from build123d import *

# Parameters (mm, degrees)
F1_W     = 76
F1_H     = 72
F2_DEPTH = 1.2
F3_R     = 30
F5_DEPTH = 28.8


with BuildPart() as f2:
    # F1 (on offset) → F2 (new body)
    with BuildSketch(Plane.XY.offset(30)):
        with Locations((0, 36)):
            Rectangle(F1_W, F1_H)
    extrude(amount=-F2_DEPTH)

    # F3
    f3_edges = [f2.edges().sort_by_distance(p)[0] for p in [
        (-38, 72, 29.4),
        (38, 72, 29.4),
    ]]
    fillet(f3_edges, radius=F3_R)

    # F4 (on face) → F5 (join, through all)
    with BuildSketch(Plane(origin=(0, 0, 28.8), x_dir=(1, 0, 0), z_dir=(0, 0, -1))):
        Polygon((5, -20), (18, -20), (18, -10), (-18, -10), (-18, -20), (-5, -20), (-5, -52), (5, -52), align=None)
        Polygon((3, -18), (3, -50), (-3, -50), (-3, -18), (-16, -18), (-16, -12), (16, -12), (16, -18), align=None, mode=Mode.SUBTRACT)
    extrude(amount=F5_DEPTH)


solid = f2.part
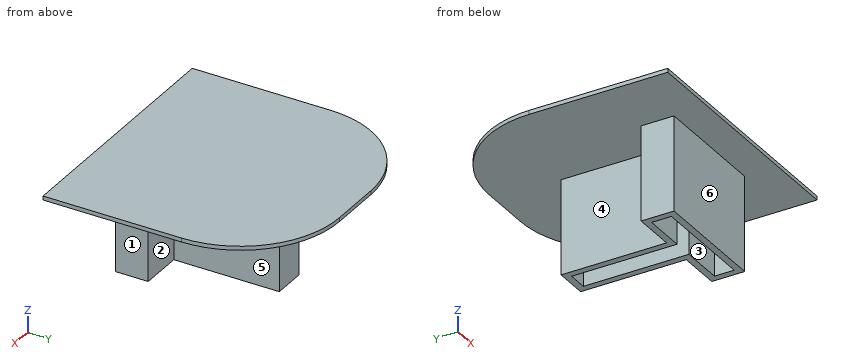
Input: part model. Units: mm. Frame: model coordinates. Face numbers are marked on the shaded views. A direction names the side the tool comes from. Give positions to 0.01 mm unless a question says otherwise; leave off trailing zeros. Order: outer loops, then holes, each group sorted by start corner. A loop starts at its lowest first (then second) coordinate and runs counter-clockwise, first axis right, second up. Notation, with made-up numbers: (29.25, 65.25) -> (60.25, 65.25) arc R6 cw to (60.25, 70.25) -> close; hole circle Ø1 at (67, 22). An arc over 180 degrees is marked (long way). Use one line per item in the form item = value.
1) Reachability of the marked faces 4, 5 and 6 from +Z, -Z, +X, -X, +Y, -Y: full face, straight path, thin tool, end or side. Return the list, or none.
Response values:
face_4 = -Z, -X, +Y
face_5 = -Z, +X, +Y
face_6 = -Z, +X, -X, -Y
2) Section A-A, the plane z = 8.75. Return loops of the section in (x, y), and give its area (3 significant figures).
Response values:
outline = (-18, 10) -> (18, 10) -> (18, 20) -> (5, 20) -> (5, 52) -> (-5, 52) -> (-5, 20) -> (-18, 20) -> close; hole (-16, 12) -> (16, 12) -> (16, 18) -> (3, 18) -> (3, 50) -> (-3, 50) -> (-3, 18) -> (-16, 18) -> close
area = 296 mm^2
3) Section C-C, the plane x = 12. Return loops of the section in (y, z).
Response values:
outline = (0, 28.8) -> (10, 28.8) -> (10, 0) -> (12, 0) -> (12, 28.8) -> (18, 28.8) -> (18, 0) -> (20, 0) -> (20, 28.8) -> (71.73, 28.8) -> (71.73, 30) -> (0, 30) -> close
4) Line query: probe 1 along X at (y, z) = (45, 7.25); probe 2 along Y at (x, z) = (5.5, 13.25); probe 3 along X at (y, z) = (17, 9.5). Output: solid intervals per line, ascending.
Response values:
probe_1 = -5 to -3, 3 to 5
probe_2 = 10 to 12, 18 to 20
probe_3 = -18 to -16, 16 to 18
5) Mould query, pull axis Y, two halves, no side actions, for the marked faces 1, 2 and 3. Classes: pulls with the +Y half, pulls with the -Y half, needs draft (parallel to the pull), parting line crosses it, or undercut.
Response values:
face_1 = needs draft
face_2 = pulls with the +Y half
face_3 = undercut
6) Section D-D, the plane x = 20. Return loops of the section in (y, z), and give its area (3 significant figures).
Response values:
outline = (0, 28.8) -> (69.5, 28.8) -> (69.5, 30) -> (0, 30) -> close
area = 83.4 mm^2
7) Section B-B, the plane y = 27. Return loops of the section in (x, z).
Response values:
outline = (-38, 28.8) -> (-5, 28.8) -> (-5, 0) -> (-3, 0) -> (-3, 28.8) -> (3, 28.8) -> (3, 0) -> (5, 0) -> (5, 28.8) -> (38, 28.8) -> (38, 30) -> (-38, 30) -> close
8) First-contact query: pin 1 Ø14.5 at (y, z) = (43.5, 13.5) entering from +X; pin 2 Ø14.5 at (x, z) = (-12, 12) entering from -Y; pin 3 Ø5 at (y, z) = (15.5, 8.5) entering from +X. Flat tips, straight axial feed; report the tip coordinate or a pass-through.
Response values:
pin_1 = 5
pin_2 = 10
pin_3 = 18
